```python
from build123d import *

# Parameters (mm, degrees)
SALIENTE_EXTRUIR1_DEPTH = 9
CROQUIS3_W              = 21
CROQUIS3_H              = 15
SALIENTE_EXTRUIR2_DEPTH = 1.5
CROQUIS4_R              = 3
CORTAR_EXTRUIR1_DEPTH   = 11.2
CROQUIS5_W              = 12
CROQUIS5_H              = 15
SALIENTE_EXTRUIR3_DEPTH = 7
CORTAR_EXTRUIR2_DEPTH   = 7
CHAFL_N1_SIZE           = 0.5
SALIENTE_EXTRUIR4_DEPTH = 1.2
CHAFL_N2_SIZE           = 1


with BuildPart() as part:
    # Croquis1 → Saliente-Extruir1 (new body)
    with BuildSketch(Plane.XY):
        with BuildLine():
            Line((-4.330127019, 2.5), (-5.2, 2.5))
            Line((-5.2, 2.5), (-5.2, -2.5))
            Line((-5.2, -2.5), (-4.330127019, -2.5))
            ThreePointArc((-4.330127019, -2.5), (-0.868240888, -4.924038765), (3.213938048, -3.830222216))
            ThreePointArc((3.213938048, -3.830222216), (5, 0), (3.213938048, 3.830222216))
            ThreePointArc((3.213938048, 3.830222216), (-0.868240888, 4.924038765), (-4.330127019, 2.5))
        make_face()
        with BuildLine():
            ThreePointArc((1.928362829, 2.298133329), (-3, 0), (1.928362829, -2.298133329))
            ThreePointArc((1.928362829, -2.298133329), (3, 0), (1.928362829, 2.298133329))
        make_face(mode=Mode.SUBTRACT)
    extrude(amount=SALIENTE_EXTRUIR1_DEPTH)

    # Croquis3 → Saliente-Extruir2 (add)
    with BuildSketch(Plane.ZY.offset(5.2)):
        with Locations((10.5, 0)):
            Rectangle(CROQUIS3_W, CROQUIS3_H)
    extrude(amount=-SALIENTE_EXTRUIR2_DEPTH)

    # Croquis4 → Cortar-Extruir1 (cut, through all)
    with BuildSketch(Plane.ZY.offset(5.2)):
        with Locations((15, 0)):
            Circle(CROQUIS4_R)
    extrude(amount=-CORTAR_EXTRUIR1_DEPTH, mode=Mode.SUBTRACT)

    # Croquis5 → Saliente-Extruir3 (add)
    with BuildSketch(Plane(origin=(-3.7, 0, 0), x_dir=(0, 0, -1), z_dir=(1, 0, 0))):
        with Locations((-15, 0)):
            Rectangle(CROQUIS5_W, CROQUIS5_H)
    extrude(amount=SALIENTE_EXTRUIR3_DEPTH)

    # Croquis7 → Cortar-Extruir2 (cut)
    with BuildSketch(Plane(origin=(3.3, 0, 0), x_dir=(0, 0, -1), z_dir=(1, 0, 0))):
        Polygon((-10, -2.886751346), (-10, 2.886751346), (-15, 5.773502692), (-20, 2.886751346), (-20, -2.886751346), (-15, -5.773502692), align=None)
    extrude(amount=-CORTAR_EXTRUIR2_DEPTH, mode=Mode.SUBTRACT)

    # Chaflán1
    chafl_n1_edges = [part.edges().sort_by_distance(p)[0] for p in [
        (-1.928362829, 2.298133329, 0),
    ]]
    chamfer(chafl_n1_edges, length=CHAFL_N1_SIZE)

    # Croquis8 → Saliente-Extruir4 (add)
    with BuildSketch(Plane(origin=(0, 7.5, 0), x_dir=(1, 0, 0), z_dir=(0, 1, 0))):
        Polygon((-3.7, 0), (3.3, -9), (-3.7, -9), align=None)
    saliente_extruir4 = extrude(amount=-SALIENTE_EXTRUIR4_DEPTH)

    # Simetría1: Saliente-Extruir4 across plane
    add(saliente_extruir4.mirror(Plane.ZX))

    # Chaflán2
    chafl_n2_edges = [part.edges().sort_by_distance(p)[0] for p in [
        (-4.45, -7.5, 0),
        (-4.45, 7.5, 0),
        (-0.95, 7.5, 21),
        (-0.95, -7.5, 21),
    ]]
    chamfer(chafl_n2_edges, length=CHAFL_N2_SIZE)


solid = part.part
```
Design review of the part built by this model. Coordinates are the model's own, in mm. A direction names the side the tool comes from. Round coordinates to 2 decimals unless told otherwise and drop trailing zeros. Write each loop counter-clockwise with the first axis right and the second up, starting at its lowest first coordinate (ties: lowest second). Pieces come first, ordered by that corner, then holes.
Item 1: We need section D-D on z = 13.5. Write out the cut boundary in (x, y).
Item 2: For faces 4 (the flat face through (-2, -6.3, 6)), 5 (the flat face through (-0.151, -4.31, 17.535)), 6 (the flat face through (4, 0, 9)), list the 3-axis set-ups (+Z, -Z, +X, -X, +Y, -Y) from which the entire face can be reached by the end or side of a thin tool; tool diameter is ignored.
Item 3: We need section C-C on x = -4. Write out the cut boundary in (y, z).
Item 4: The part is to be moulded in two halves that separate along Z. For faces 1 (the flat face through (0, 0, 10)), 2 (the flat face through (-1, 0, 21)), 3 (the flat face through (3.3, 0.1, 20.4)), say which applies: +Z half, -Z half, draft (parallel to the pull), parting line (faces both ways), or undercut.
Item 5: Clearance check with flat-ended pins moving along their axes: pin 1 Ø8 at (y, z) = (2, 15.5) entering from +X; pin 2 Ø2 at (x, y) = (3.5, -2) entering from +Z; pin 3 Ø3 at (y, z) = (-5.5, 6.5) entering from +X; pin 4 Ø0.9 at (x, y) = (4.5, -0.5) entering from +Z. State where each tip first meets the part, or that it passes through.
Item 6: For probe 1 along Y at (x, z) = (0, 7.25); probe 2 along Y at (x, z) = (-4.6, 15); probe 3 along Z at (x, y) = (0.5, 2.75), list the stretches that pass through material, from the lowest coordinate up.
Item 7: We need section B-B on z = 17.25. Write out the cut boundary in (x, y).
Item 8: We need section A-A on y = 0. Write out the cut boundary in (x, z), and give its area (4 significant figures).
Returned:
1. outline: (-5.2, -7.5) - (3.3, -7.5) - (3.3, -4.91) - (-3.7, -4.91) - (-3.7, -2.6) - (-5.2, -2.6) - close; (-5.2, 2.6) - (-3.7, 2.6) - (-3.7, 4.91) - (3.3, 4.91) - (3.3, 7.5) - (-5.2, 7.5) - close
2. face 4: -Z, +X
2. face 5: +X
2. face 6: +Z, +X, +Y, -Y
3. outline: (-7.5, 1) - (-6.5, 0) - (6.5, 0) - (7.5, 1) - (7.5, 20) - (6.5, 21) - (-6.5, 21) - (-7.5, 20) - close; hole circle Ø6 at (0, 15)
4. face 1: undercut
4. face 2: +Z half
4. face 3: draft
5. pin 1: stops at x = 3.3
5. pin 2: stops at z = 21
5. pin 3: stops at x = 3
5. pin 4: stops at z = 9
6. probe 1: y = -7.5 to -6.3, -5 to -3, 3 to 5, 6.3 to 7.5
6. probe 2: y = -7.5 to -3, 3 to 7.5
6. probe 3: z = 9 to 10, 20 to 21
7. outline: (-5.2, -7.5) - (3.3, -7.5) - (3.3, -4.47) - (-3.7, -4.47) - (-3.7, -1.98) - (-5.2, -1.98) - close; (-5.2, 1.98) - (-3.7, 1.98) - (-3.7, 4.47) - (3.3, 4.47) - (3.3, 7.5) - (-5.2, 7.5) - close
8. outline: (-5.2, 0) - (-3.5, 0) - (-3, 0.5) - (-3, 9) - (3, 9) - (3, 0.5) - (3.5, 0) - (5, 0) - (5, 9) - (3.3, 9) - (3.3, 10) - (-3.7, 10) - (-3.7, 12) - (-5.2, 12) - close; (-5.2, 18) - (-3.7, 18) - (-3.7, 20) - (3.3, 20) - (3.3, 21) - (-5.2, 21) - close
8. area: 60.55 mm2
